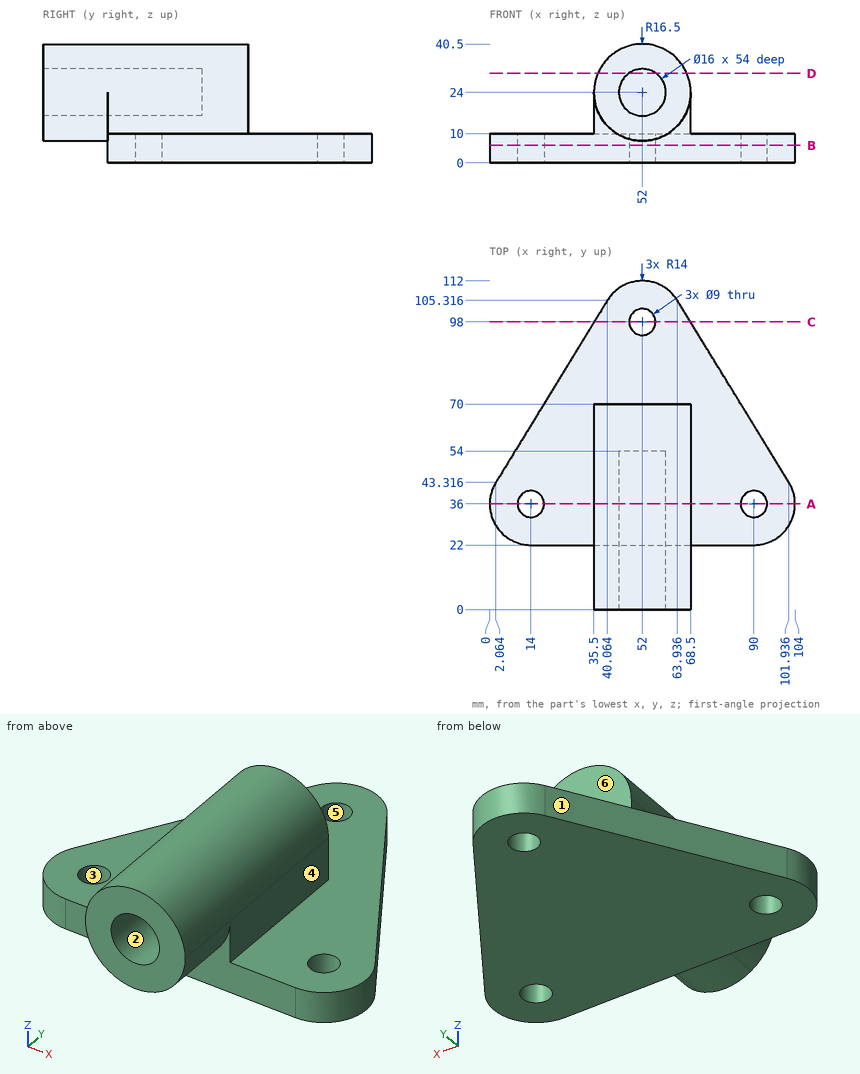
Here's the drawing with two shaded views (mm, measured from the low corner). I have some questions. A direction names the side the tool comes from. Coordinates: 2 decimals unless noted, no trailing zeros. Order: outer loops, then holes, each group sorted by start corner. A loop starts at its lowest first (then second) coordinate and runs counter-clockwise, first axis right, second up. Notation, with made-up numbers: (-29.5, 12) - (26.5, 12) arc R21 cw to (26.5, 21) - close; hole circle Ø3 at (-21, -11.5). An arc over 180 degrees is marked (long way). Answer in a Markdown table with one row per item. Add a question column.
(1) If we section it at C-C, the plane y = 98: Please give me the cut outline in (x, z), then the cut area to 3 significant figures.
(2) If we section it at D-D, the plane z = 30.5: Please give me the cut outline in (x, y) (1 decimal).
(3) On a 3-axis mill with a long thin cutter (end or side, diameter ignored), from which of +Z, -Z, +X, -X, +Y, -Y can I reach the whole of each face in a straight line? I mean the marked faces 4, 5 and 6. Say none if no direction works.
(4) If we section it at A-A, the plane y = 36: Please give me the cut outline in (x, z), then the cut area to 3 significant figures.
(5) If we mould it in two halves opening along Y, with no side actions, what happens to the marked faces 1, 2 and 3? For each: released by +Y, released by -Y, zero draft, split by the parting line, or undercut.
(6) Will these pins go through, and if not, where does the flat tip stop? pin 1 (4 mm diameter, centred on y = 36.5, z = 15.5, fed in from +X); pin 2 (12 mm diameter, centred on x = 42.5, y = 66, fed in from -Z); pin 3 (9 mm diameter, centred on x = 50.5, z = 25, fed in from +Y); pin 4 (8 mm diameter, centred on x = 29, y = 69, fed in from +Z).
(7) I need wall thicknesses on L1, parallel to Y at x = 52, z = 5.25; L2, parallel to Z at x = 52, y = 26; L3, parallel to Y at x = 90, z = 4.5. Which ranges of each line are inside material? Lowest first, please.
(8) If we section it at B-B, the plane z = 6: Please give me the cut outline in (x, y), then the cut area to 3 significant figures.
Results are:
| question | item | result |
|---|---|---|
| 1 | outline | (35.58, 0) - (47.5, 0) - (47.5, 10) - (35.58, 10) - close; (56.5, 0) - (68.42, 0) - (68.42, 10) - (56.5, 10) - close |
| 1 | area | 238 mm2 |
| 2 | outline | (36.8, 0) - (47.3, 0) - (47.3, 54) - (56.7, 54) - (56.7, 0) - (67.2, 0) - (67.2, 70) - (36.8, 70) - close |
| 3 | face 4 | +Z, +X, +Y, -Y |
| 3 | face 5 | +Z, -Z |
| 3 | face 6 | +Z, +X, -X, +Y |
| 4 | outline | (0, 0) - (9.5, 0) - (9.5, 10) - (0, 10) - close; (18.5, 0) - (85.5, 0) - (85.5, 10) - (68.5, 10) - (68.5, 24) arc R16.5 ccw to (35.5, 24) - (35.5, 10) - (18.5, 10) - close; (94.5, 0) - (104, 0) - (104, 10) - (94.5, 10) - close; hole circle Ø16 at (52, 24) |
| 4 | area | 1,550 mm2 |
| 5 | face 1 | released by +Y |
| 5 | face 2 | zero draft |
| 5 | face 3 | undercut |
| 6 | pin 1 | stops at x = 68.5 |
| 6 | pin 2 | stops at z = 0 |
| 6 | pin 3 | stops at y = 70 |
| 6 | pin 4 | stops at z = 10 |
| 7 | L1 | y = 22 to 93.5, 102.5 to 112 |
| 7 | L2 | z = 0 to 16, 32 to 40.5 |
| 7 | L3 | y = 22 to 31.5, 40.5 to 62.79 |
| 8 | outline | (2.06, 43.32) arc R14 ccw to (14, 22) - (90, 22) arc R14 ccw to (101.94, 43.32) - (63.94, 105.32) arc R14 ccw to (40.06, 105.32) - close; hole circle Ø9 at (14, 36); hole circle Ø9 at (52, 98); hole circle Ø9 at (90, 36) |
| 8 | area | 5,880 mm2 |
